Model file for the job. Use its own axes, mm. A direction names the side the tool comes from. Round coordinates to 2 decimals unless told otherwise and drop trailing zeros. Loops run counter-clockwise (first coordinate to the right, second up) from the corner with the lowest first, then second, coordinate; pieces in that order, holes last. Notation, with made-up numbers: M 25,69 L 38,69 A33 cw 38,101 Z; hole C 42.5,68.5 d2. An arc over 180 degrees is marked long. Use a Markdown table: item, result. Add a question column.
Q1. Mould opens along Y. For faces 1 (the face through (0, 84, 0)), 2 (the face through (14.048, 76.419, 14.895)), 3 (the face through (0.602, 57.944, 2.713)), 4 (the face through (-10.952, 76.419, 14.895)) say: +Y half, -Y half, draft (parallel to the pull), parting line (faces both ways), or undercut.
Q2. Probe line 1 (X direction, y = 75, z = 10.5); line 2 (Y direction, x = 12.5, z = 20); line 3 (Z direction, x = -6.5, y = 11.5). List the from-to ranges inside material, lowest first. Write a range as from..to.
Q3. Pin check, flat tips, straight feed: pin 1 (2.5 mm diameter, centred on x = -12.5, y = 75, fed in from +Z); pin 2 (8 mm diameter, centred on x = 10, y = 125, fed in from -Z); pin 3 (4 mm diameter, centred on x = 2.5, z = 12, fed in from +Y). Stop position of each tip, or through.
Q4. Cut at A-A (y = 22). Give the cut face in (x, z), plus the area to 3 significant figures.
Q5. Cut at B-B (y = 107). Give the cut face in (x, z), plus the area to 3 significant figures.
Q6. Tool access for faces 5 (the face through (0, 130, 3)), 6 (the face through (0, 75, -17.5)), 7 (the face through (12.96, 110.95, 17.43)), 8 (the face through (0, 35, -22.5)), 9 (the face through (-14.048, 76.419, -12.43)): list every direction of +Z, -Z, +X, -X, +Y, -Y with a clear straight run to the whole face (end or side of a thin tool).
from build123d import *

# Parameters (mm, degrees)
SKETCH_1_W                       = 45
SKETCH_1_H                       = 45
EXTRUDE_1_DEPTH                  = 80
HOLE_WIZARD_M36_1_D              = 32
HOLE_WIZARD_M36_1_DEPTH          = 50
HOLE_WIZARD_M36_1_CSINK_D        = 38
HOLE_WIZARD_M36_1_CSINK_ANGLE    = 90
HOLE_WIZARD_M36_1_TIP            = 9.613769904
SKETCH_6_W                       = 5
SKETCH_6_H                       = 10
EXTRUDE_2_DEPTH                  = 45
SKETCH_7_R                       = 2.5
CUT_EXTRUDE_1_DEPTH              = 135.768319719
SKETCH_8_W                       = 5
SKETCH_8_H                       = 10
CUT_EXTRUDE_2_DEPTH              = 140.396018595
HOLE_WIZARD_M5_1_D               = 4.2
HOLE_WIZARD_M5_1_DEPTH           = 15
HOLE_WIZARD_M5_1_TIP             = 1.2618073
HOLE_WIZARD_M5_2_D               = 4.2
HOLE_WIZARD_M5_2_DEPTH           = 10
HOLE_WIZARD_M5_2_TIP             = 1.2618073
HOLE_WIZARD_M5_2_ON_FACE_2_D     = 4.2
HOLE_WIZARD_M5_2_ON_FACE_2_DEPTH = 10
HOLE_WIZARD_M5_2_ON_FACE_2_TIP   = 1.2618073


with BuildPart() as part:
    # 草图1 → 凸台-拉伸1 (new body)
    with BuildSketch(Plane(origin=(0, 0, 0), x_dir=(1, 0, 0), z_dir=(0, 1, 0))):
        Rectangle(SKETCH_1_W, SKETCH_1_H)
    extrude(amount=EXTRUDE_1_DEPTH)

    # M36 螺纹孔1
    with Locations(Plane(origin=(0, 0, 0), x_dir=(-1, 0, 0), z_dir=(0, -1, 0))):
        with Locations((0, 0)):
            CounterSinkHole(HOLE_WIZARD_M36_1_D / 2, HOLE_WIZARD_M36_1_CSINK_D / 2, depth=HOLE_WIZARD_M36_1_DEPTH, counter_sink_angle=HOLE_WIZARD_M36_1_CSINK_ANGLE)
            with Locations((0, 0, -(HOLE_WIZARD_M36_1_DEPTH + HOLE_WIZARD_M36_1_TIP / 2))):  # 118° drill point
                Cone(0, HOLE_WIZARD_M36_1_D / 2, HOLE_WIZARD_M36_1_TIP, mode=Mode.SUBTRACT)

    # 草图6 → 凸台-拉伸2 (add)
    with BuildSketch(Plane(origin=(22.5, 0, 0), x_dir=(0, 0, -1), z_dir=(1, 0, 0))):
        with BuildLine():
            Line((-22.5, 100), (-22.5, 80))
            Line((-22.5, 80), (0, 80))
            Line((0, 80), (0, 88))
            ThreePointArc((0, 88), (-8.485281374, 91.514718626), (-12, 100))
            Line((-12, 100), (-22.5, 100))
        make_face()
        with BuildLine():
            Line((-22.5, 120), (-22.5, 100))
            Line((-22.5, 100), (-12, 100))
            ThreePointArc((-12, 100), (-8.485281374, 108.485281374), (0, 112))
            Line((0, 112), (0, 120))
            Line((0, 120), (-5, 120))
            Line((-5, 120), (-22.5, 120))
        make_face()
        with Locations((-2.5, 125)):
            Rectangle(SKETCH_6_W, SKETCH_6_H)
    extrude(amount=-EXTRUDE_2_DEPTH)

    # 草图7 → 切除-拉伸1 (cut, through all)
    with BuildSketch(Plane.XY.offset(5)):
        with Locations((10, 125)):
            Circle(SKETCH_7_R)
        with Locations((-10, 125)):
            Circle(SKETCH_7_R)
    extrude(amount=-CUT_EXTRUDE_1_DEPTH, mode=Mode.SUBTRACT)

    # 草图8 → 切除-拉伸2 (cut, through all)
    with BuildSketch(Plane(origin=(22.5, 0, 0), x_dir=(0, 0, -1), z_dir=(1, 0, 0))):
        with Locations((20, 75)):
            Rectangle(SKETCH_8_W, SKETCH_8_H)
    extrude(amount=-CUT_EXTRUDE_2_DEPTH, mode=Mode.SUBTRACT)

    # M5 螺纹孔的螺纹孔钻头1
    with Locations(Plane(origin=(-12.5, 75, 22.5), x_dir=(1, 0, 0), z_dir=(0, 0, 1))):
        with Locations((0, 0), (25, 0)):
            Hole(HOLE_WIZARD_M5_1_D / 2, depth=HOLE_WIZARD_M5_1_DEPTH)
            with Locations((0, 0, -(HOLE_WIZARD_M5_1_DEPTH + HOLE_WIZARD_M5_1_TIP / 2))):  # 118° drill point
                Cone(0, HOLE_WIZARD_M5_1_D / 2, HOLE_WIZARD_M5_1_TIP, mode=Mode.SUBTRACT)

    # M5 螺纹孔的螺纹孔钻头2
    with Locations(Plane(origin=(12.5, 75, -17.5), x_dir=(-1, 0, 0), z_dir=(0, 0, -1))):
        with Locations((0, 0), (25, 0)):
            Hole(HOLE_WIZARD_M5_2_D / 2, depth=HOLE_WIZARD_M5_2_DEPTH)
            with Locations((0, 0, -(HOLE_WIZARD_M5_2_DEPTH + HOLE_WIZARD_M5_2_TIP / 2))):  # 118° drill point
                Cone(0, HOLE_WIZARD_M5_2_D / 2, HOLE_WIZARD_M5_2_TIP, mode=Mode.SUBTRACT)

    # M5 螺纹孔的螺纹孔钻头2 on face 2
    with Locations(Plane(origin=(-12.5, 113, 22.5), x_dir=(1, 0, 0), z_dir=(0, 0, 1))):
        with Locations((0, 0), (25, 0)):
            Hole(HOLE_WIZARD_M5_2_ON_FACE_2_D / 2, depth=HOLE_WIZARD_M5_2_ON_FACE_2_DEPTH)
            with Locations((0, 0, -(HOLE_WIZARD_M5_2_ON_FACE_2_DEPTH + HOLE_WIZARD_M5_2_ON_FACE_2_TIP / 2))):  # 118° drill point
                Cone(0, HOLE_WIZARD_M5_2_ON_FACE_2_D / 2, HOLE_WIZARD_M5_2_ON_FACE_2_TIP, mode=Mode.SUBTRACT)


solid = part.part
Checked values:
| question | item | result |
|---|---|---|
| 1 | face 1 | draft |
| 1 | face 2 | undercut |
| 1 | face 3 | -Y half |
| 1 | face 4 | undercut |
| 2 | line 1 | x = -22.5..-14.6, -10.4..10.4, 14.6..22.5 |
| 2 | line 2 | y = 0..72.9, 77.1..110.9, 115.1..120 |
| 2 | line 3 | z = -22.5..-14.62, 14.62..22.5 |
| 3 | pin 1 | stops at z = 6.99 |
| 3 | pin 2 | stops at z = 0 |
| 3 | pin 3 | stops at y = 120 |
| 4 | outline | M -22.5,-22.5 L 22.5,-22.5 L 22.5,22.5 L -22.5,22.5 Z; hole C 0,0 d32 |
| 4 | area | 1,220 mm^2 |
| 5 | outline | M -22.5,9.75 L 22.5,9.75 L 22.5,22.5 L -22.5,22.5 Z |
| 5 | area | 574 mm^2 |
| 6 | face 5 | +Z, -Z, +X, -X, +Y |
| 6 | face 6 | -Z, +X, -X, +Y |
| 6 | face 7 | +Z |
| 6 | face 8 | -Z, +X, -X, +Y, -Y |
| 6 | face 9 | -Z |
